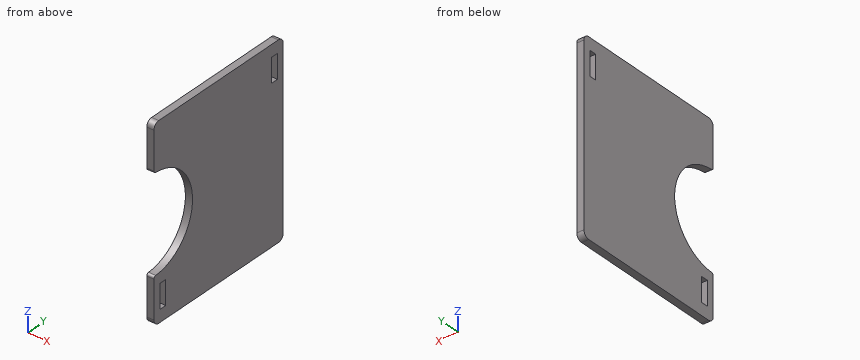
```python
from build123d import *

# Parameters (mm, degrees)
SALIENTE_EXTRUIR1_DEPTH = 3
CROQUIS2_R              = 20
CROQUIS2_W              = 10.1
CROQUIS2_H              = 3.1
CORTAR_EXTRUIR1_DEPTH   = 3
REDONDEO1_R             = 1


with BuildPart() as part:
    # Croquis1 → Saliente-Extruir1 (new body)
    with BuildSketch(Plane(origin=(0, 0, 0), x_dir=(0, 0, -1), z_dir=(1, 0, 0))):
        with BuildLine():
            Line((-36.82, 33.5), (36.82, 33.5))
            ThreePointArc((36.82, 33.5), (38.587766953, 32.767766953), (39.32, 31))
            Line((39.32, 31), (39.32, -31))
            ThreePointArc((39.32, -31), (38.587766953, -32.767766953), (36.82, -33.5))
            Line((36.82, -33.5), (-36.82, -33.5))
            ThreePointArc((-36.82, -33.5), (-38.587766953, -32.767766953), (-39.32, -31))
            Line((-39.32, -31), (-39.32, 31))
            ThreePointArc((-39.32, 31), (-38.587766953, 32.767766953), (-36.82, 33.5))
        make_face()
    extrude(amount=SALIENTE_EXTRUIR1_DEPTH)

    # Croquis2 → Cortar-Extruir1 (cut, symmetric)
    with BuildSketch(Plane(origin=(3, 0, 0), x_dir=(0, 0, -1), z_dir=(1, 0, 0))):
        with Locations((0, -33.5)):
            Circle(CROQUIS2_R)
        with Locations((29.18492387, -28.95)):
            Rectangle(CROQUIS2_W, CROQUIS2_H)
        with Locations((-29.32, 28.95)):
            Rectangle(CROQUIS2_W, CROQUIS2_H)
    extrude(amount=CORTAR_EXTRUIR1_DEPTH, both=True, mode=Mode.SUBTRACT)

    # Redondeo1
    redondeo1_edges = [part.edges().sort_by_distance(p)[0] for p in [
        (1.5, -33.5, 20),
        (1.5, -33.5, -20),
    ]]
    fillet(redondeo1_edges, radius=REDONDEO1_R)


solid = part.part
```
The model under review builds one solid part; all positions refer to its coordinate system, in mm. Coordinates: 2 decimals unless noted, no trailing zeros. Write each loop counter-clockwise with the first axis right and the second up, starting at its lowest first coordinate (ties: lowest second). Pieces come first, ordered by that corner, then holes. Notation, with made-up numbers: (-26, -30) - (17, -30) arc R35 cw to (17, 2) - close; hole circle Ø9 at (-21.5, 31.25). An arc over 180 degrees is marked (long way). Write item = value, one per line.
(1) Consider section B-B, the plane y = -26.5. Give the boundary of the cut face in (x, z) (3 decimals).
Result sheet:
outline = (0, -39.32) - (3, -39.32) - (3, -18.735) - (0, -18.735) - close; (0, 18.735) - (3, 18.735) - (3, 39.32) - (0, 39.32) - close
(2) Consider section A-A, the plane z = -25.5. Give the boundary of the cut face in (x, y).
Result sheet:
outline = (0, -33.5) - (3, -33.5) - (3, -30.5) - (0, -30.5) - close; (0, -27.4) - (3, -27.4) - (3, 33.5) - (0, 33.5) - close
(3) Consider section C-C, the plane x = 1.6. Give the boundary of the cut face in (y, z).
Result sheet:
outline = (-33.5, -36.82) arc R2.5 ccw to (-31, -39.32) - (31, -39.32) arc R2.5 ccw to (33.5, -36.82) - (33.5, 36.82) arc R2.5 ccw to (31, 39.32) - (-31, 39.32) arc R2.5 ccw to (-33.5, 36.82) - (-33.5, 20.98) arc R1 ccw to (-32.55, 19.98) arc R20 cw to (-32.55, -19.98) arc R1 ccw to (-33.5, -20.98) - close; hole (-30.5, -34.23) - (-27.4, -34.23) - (-27.4, -24.13) - (-30.5, -24.13) - close; hole (27.4, 24.27) - (30.5, 24.27) - (30.5, 34.37) - (27.4, 34.37) - close
(4) For P1, Ø1, axis at x = 2, z = -8, coming from the -Y side, flat-tipped, find the tip position at first contact; note if it passes through.
Result sheet:
P1 = -15.4
(5) Consider section D-D, the plane z = 0. Give the boundary of the cut face in (x, y), then the cut area to 3 significant figures.
Result sheet:
outline = (0, -13.5) - (3, -13.5) - (3, 33.5) - (0, 33.5) - close
area = 141 mm^2
(6) For line 1 (Y direction, x = 2.25, z = 29.5); line 2 (Y direction, x = 0.25, z = -33); line 3 (Y direction, x = 2.05, z = 0.5), list the stretches that pass through material, from the lowest coordinate up. Write a range as [from, to].
Result sheet:
line_1 = [-33.5, 27.4], [30.5, 33.5]
line_2 = [-33.5, -30.5], [-27.4, 33.5]
line_3 = [-13.51, 33.5]
